Design review of the part built by this model. Coordinates are the model's own, in mm. Face numbers are marked on the shaded views. A direction names the side the tool comes from. Round coordinates to 2 decimals unless told otherwise and drop trailing zeros. Write each loop counter-clockwise with the first axis right and the second up, starting at its lowest first coordinate (ties: lowest second). Pieces come first, ordered by that corner, then holes. Notation, with made-up numbers: (30.5, 72) - (55.5, 72) arc R12 ccw to (55.5, 82) - close; hole circle Ø3 at (-23.5, 36.25). An arc over 180 degrees is marked (long way). Use one line per item in the form item = value.
```python
from build123d import *

# Parameters (mm, degrees)
SKETCH1_R           = 32.004
BOSS_EXTRUDE1_DEPTH = 114.6048
SKETCH2_R           = 32.004
SKETCH2_R_2         = 15.0368
CUT_EXTRUDE1_DEPTH  = 5.0038
SKETCH3_R           = 2.0193
CUT_EXTRUDE2_DEPTH  = 13.6144
SKETCH4_R           = 9.525
BOSS_EXTRUDE2_DEPTH = 3.9878
SKETCH6_R           = 4.0005
BOSS_EXTRUDE3_DEPTH = 35.6108


with BuildPart() as part:
    # Sketch1 → Boss-Extrude1 (new body)
    with BuildSketch(Plane(origin=(0, 0, 0), x_dir=(1, 0, 0), z_dir=(0, 1, 0))):
        Circle(SKETCH1_R)
    extrude(amount=BOSS_EXTRUDE1_DEPTH)

    # Sketch2 → Cut-Extrude1 (cut)
    with BuildSketch(Plane(origin=(0, 114.6048, 0), x_dir=(1, 0, 0), z_dir=(0, 1, 0))):
        Circle(SKETCH2_R)
        Circle(SKETCH2_R_2, mode=Mode.SUBTRACT)
    extrude(amount=-CUT_EXTRUDE1_DEPTH, mode=Mode.SUBTRACT)

    # Sketch3 → Cut-Extrude2 (cut)
    with BuildSketch(Plane(origin=(0, 0, 0), x_dir=(-1, 0, 0), z_dir=(0, -1, 0))):
        with Locations((0, -25.4)):
            Circle(SKETCH3_R)
        with Locations((0, 25.4)):
            Circle(SKETCH3_R)
    extrude(amount=-CUT_EXTRUDE2_DEPTH, mode=Mode.SUBTRACT)

    # Sketch4 → Boss-Extrude2 (add)
    with BuildSketch(Plane.XZ):
        Circle(SKETCH4_R)
    extrude(amount=BOSS_EXTRUDE2_DEPTH)

    # Sketch6 → Boss-Extrude3 (add)
    with BuildSketch(Plane(origin=(0, 0, 0), x_dir=(-1, 0, 0), z_dir=(0, -1, 0))):
        Circle(SKETCH6_R)
    extrude(amount=BOSS_EXTRUDE3_DEPTH)


solid = part.part
```
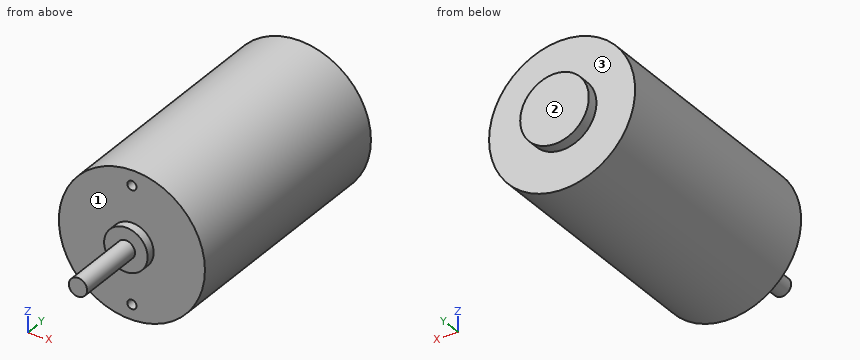
Q1. We need section D-D on y = 87. Write out the cut boundary in (x, z), then the cut area to 3 significant figures.
Calculated:
outline = circle Ø64.01 at (0, 0)
area = 3,220 mm2
Q2. We need section B-B on x = 0. Write out the cut boundary in (y, z) (1 decimal).
Calculated:
outline = (-35.6, -4) - (-4, -4) - (-4, -9.5) - (0, -9.5) - (0, -23.4) - (13.6, -23.4) - (13.6, -27.4) - (0, -27.4) - (0, -32) - (109.6, -32) - (109.6, -15) - (114.6, -15) - (114.6, 15) - (109.6, 15) - (109.6, 32) - (0, 32) - (0, 27.4) - (13.6, 27.4) - (13.6, 23.4) - (0, 23.4) - (0, 9.5) - (-4, 9.5) - (-4, 4) - (-35.6, 4) - close
Q3. To check wall thickness, follow line 1 along Z through (x, y) = (0, 10); line 2 along Y through (x, z) = (13, 5); line 3 along Y through (x, z) = (-6.5, 1.5). State the ranges of each line that lie inside material, in increasing order. Write a range as from..to.
Calculated:
line_1 = -32..-27.42, -23.38..23.38, 27.42..32
line_2 = 0..114.6
line_3 = -3.99..114.6
Q4. We need section A-A on z = 0. Write out the cut boundary in (x, y) (1 decimal).
Calculated:
outline = (-32, 0) - (-9.5, 0) - (-9.5, -4) - (-4, -4) - (-4, -35.6) - (4, -35.6) - (4, -4) - (9.5, -4) - (9.5, 0) - (32, 0) - (32, 109.6) - (15, 109.6) - (15, 114.6) - (-15, 114.6) - (-15, 109.6) - (-32, 109.6) - close
Q5. We need section C-C on y = 12. Write out the cut boundary in (x, z), then the cut area to 3 significant figures.
Calculated:
outline = circle Ø64.01 at (0, 0); hole circle Ø4.04 at (0, -25.4); hole circle Ø4.04 at (0, 25.4)
area = 3,190 mm2
Q6. For P1, Ø2.5, axis at x = 0, z = -25.4, coming from the -Y side; P2, Ø10, axis at x = 12, z = -3.5, coming from the -Y side; P3, Ø4, axis at x = 24.5, z = 16, coming from the -Y side, all flat-tipped, find the tip position at first contact; note any pin that passes through.
Calculated:
P1 = 13.61
P2 = -3.99
P3 = 0
Q7. Machinability: for the marked faces 1, 2 and 3, which of the approach directions +Z, -Z, +X, -X, +Y, -Y give a long, thin tool a straight path to every point of the face, cutting with its end or side? Answer none if there is none.
Calculated:
face_1 = -Y
face_2 = +Z, -Z, +X, -X, +Y
face_3 = +Y
